from build123d import *

# Parameters (mm, degrees)
F0_W     = 90
F0_H     = 300
F1_DEPTH = 40
F2_R     = 10
F3_T     = -4


# Not quite as in the source:
# - a shell that OpenCascade refuses in one call is made with other operations: the cavity is built on its own and cut out


with BuildPart() as f1:
    # F0 (on Top) → F1 (new body)
    with BuildSketch(Plane.XY):
        with Locations((-168.3901532187, 84.1299444437)):
            Rectangle(F0_W, F0_H)
    extrude(amount=F1_DEPTH)

    # F2
    f2_edges = [f1.edges().sort_by_distance(p)[0] for p in [
        (-123.390153, 84.129944, 40),
        (-168.390153, -65.870056, 40),
        (-213.390153, 84.129944, 40),
        (-168.390153, 234.129944, 40),
        (-168.390153, -65.870056, 0),
        (-123.390153, 84.129944, 0),
        (-123.390153, 234.129944, 20),
        (-123.390153, -65.870056, 20),
        (-213.390153, -65.870056, 20),
        (-213.390153, 234.129944, 20),
        (-213.390153, 84.129944, 0),
        (-168.390153, 234.129944, 0),
    ]]
    fillet(f2_edges, radius=F2_R)

    # F3: a shell. OpenCascade refuses it in one call, so the cavity is built on its own and cut out:
    # the body offset inwards by the wall thickness, plus a prism from it out through each open face.
    f3_core = offset(f1.part, amount=F3_T, mode=Mode.PRIVATE)
    f3_exits = [f3_core.faces().sort_by_distance(p)[0] for p in [
        (-168.390153, 84.129944, 36),
    ]]
    add(f3_core, mode=Mode.SUBTRACT)
    extrude(f3_exits, amount=-F3_T, mode=Mode.SUBTRACT)


solid = f1.part
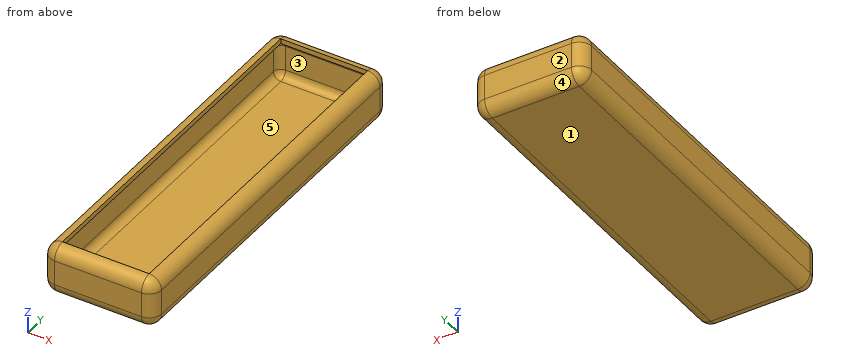
Read the model definition and answer for the solid it produces. Units are mm, in the model's axes. Face numbers are marked on the shaded views. A direction names the side the tool comes from. Give positions to 0.01 mm unless a question says otherwise; leave off trailing zeros. Write each loop counter-clockwise with the first axis right and the second up, starting at its lowest first coordinate (ties: lowest second). Pieces come first, ordered by that corner, then holes. Notation, with made-up numbers: (70, -37) - (79, -37) arc R18 ccw to (79, -5) - close; hole circle Ø1 at (5.5, 40.25). An arc over 180 degrees is marked (long way). Answer in a Markdown table with one row per item. Add a question column.
Item 1: Section B-B, the plane y = -7 is taken. Write down the section's boundary in (x, z).
Item 2: Section C-C, the plane x = -167.5 is taken. Write down the section's boundary in (y, z).
Item 3: Section A-A, the plane z = 21 is taken. Write down the section's boundary in (x, y).
Item 4: A tool of negligible diameter and unlimited length cuts with its end or side. For the marked faces 4 and 5, from which of +Z, -Z, +X, -X, +Y, -Y can it reach the whole face along a straight path? Write none if from no direction.
Item 5: Flat-ended cylindrical pins translate along their axes: P1, Ø3, axis at y = 138, z = 37, coming from the -X side; P2, Ø4.5, axis at y = 114, z = 37.5, coming from the +X side; P3, Ø1.5, axis at y = 26.5, z = 33.5, coming from the +X side. Find the tip coordinate at first contact, or state that the pin passes through.
Item 6: Find the intervals of material crossed by L1, parallel to Y at x = -188.5, z = 19.5; L2, parallel to X at y = 196, z = 26; L3, parallel to Z at x = -162, y = 38.5, in increasing order.
Item 7: Determine the mould class of the marked faces 1, 2 and 3 for opening direction Z: pulls with the +Z half, pulls with the -Z half, needs draft (parallel to the pull), parting line crosses it, or undercut.
Recorded:
| question | item | result |
|---|---|---|
| 1 | outline | (-213.39, 10) arc R10 ccw to (-203.39, 0) - (-133.39, 0) arc R10 ccw to (-123.39, 10) - (-123.39, 30) arc R10 ccw to (-133.39, 40) - (-133.39, 36) arc R6 cw to (-127.39, 30) - (-127.39, 10) arc R6 cw to (-133.39, 4) - (-203.39, 4) arc R6 cw to (-209.39, 10) - (-209.39, 30) arc R6 cw to (-203.39, 36) - (-203.39, 40) arc R10 ccw to (-213.39, 30) - close |
| 2 | outline | (-65.87, 10) arc R10 ccw to (-55.87, 0) - (224.13, 0) arc R10 ccw to (234.13, 10) - (234.13, 30) arc R10 ccw to (224.13, 40) - (224.13, 36) arc R6 cw to (230.13, 30) - (230.13, 10) arc R6 cw to (224.13, 4) - (-55.87, 4) arc R6 cw to (-61.87, 10) - (-61.87, 30) arc R6 cw to (-55.87, 36) - (-55.87, 40) arc R10 ccw to (-65.87, 30) - close |
| 3 | outline | (-213.39, -55.87) arc R10 ccw to (-203.39, -65.87) - (-133.39, -65.87) arc R10 ccw to (-123.39, -55.87) - (-123.39, 224.13) arc R10 ccw to (-133.39, 234.13) - (-203.39, 234.13) arc R10 ccw to (-213.39, 224.13) - close; hole (-209.39, -55.87) arc R6 ccw to (-203.39, -61.87) - (-133.39, -61.87) arc R6 ccw to (-127.39, -55.87) - (-127.39, 224.13) arc R6 ccw to (-133.39, 230.13) - (-203.39, 230.13) arc R6 ccw to (-209.39, 224.13) - close |
| 4 | face 4 | -Z, +X, -X, +Y |
| 4 | face 5 | +Z |
| 5 | P1 | stops at x = -211.74 |
| 5 | P2 | stops at x = -124.88 |
| 5 | P3 | stops at x = -123.78 |
| 6 | L1 | y = -65.87 to -61.87, 230.13 to 234.13 |
| 6 | L2 | x = -213.39 to -209.39, -127.39 to -123.39 |
| 6 | L3 | z = 0 to 4 |
| 7 | face 1 | pulls with the -Z half |
| 7 | face 2 | needs draft |
| 7 | face 3 | undercut |
